Autodesk Inventor part; units mm, degrees
ref_plane "YZ Plane" through (0, 0, 0) normal (1, 0, 0) x (0, 1, 0)
ref_plane "XZ Plane" through (0, 0, 0) normal (0, 1, 0) x (-1, 0, 0)
ref_plane "XY Plane" through (0, 0, 0) normal (0, 0, 1) x (1, 0, 0)
sketch "Sketch1" plane through (0, 0, 0) normal (0, 1, 0) x (-1, 0, 0)
  circle A0 centre (0, 0) radius 12.5
  dimension "d0" = 25
extrude "Extrusion1" add sketch "Sketch1" along normal blind 1
sketch "Sketch2" plane through (0, 1, 0) normal (0, 1, 0) x (1, 0, 0)
  circle A0 centre (0, 0) radius 9.5
  dimension "d3" = 19
extrude "Extrusion2" add sketch "Sketch2" along normal blind 5
sketch "Sketch3" plane through (0, 6, 0) normal (0, 1, 0) x (1, 0, 0)
  circle A0 centre (0, 0) radius 12.5
  dimension "d6" = 25
extrude "Extrusion3" add sketch "Sketch3" along normal blind 1
hole "Hole1" at (-6.2494, 7, 8.9167) direction (0, -1, 0) diameter 1 depth 7
sketch "Sketch4" plane through (0, 7, 0) normal (0, 1, 0) x (1, 0, 0)
  circle A0 centre (0, 0) radius 8.5
  dimension "d18" = 17
extrude "Extrusion4" cut sketch "Sketch4" against normal blind 7
thread "Thread1"
sketch "Sketch5" plane through (0, 0, 0) normal (0, -1, 0) x (1, 0, 0)
  line L0 (11.3779, 4.9373) -> (8.8779, 4.9373)
  line L1 (8.8779, 4.9373) -> (8.8779, -5.0627)
  line L2 (8.8779, -5.0627) -> (11.3779, -5.0627)
  line L3 (11.3779, -5.0627) -> (11.3779, 4.9373)
  point P0 (0, 0)
  dimension "d23" = 10
  dimension "d24" = 2.5
extrude "Extrusion5" add sketch "Sketch5" along normal blind 10
properties part number "Ttube1"
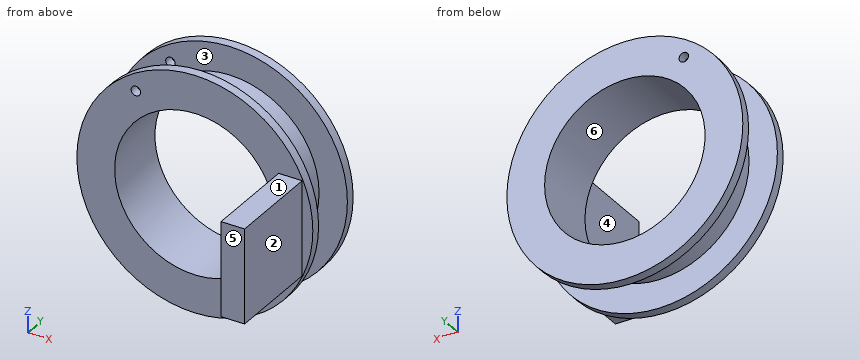
Source: CAD feature listing. Evaluate the final solid. Frame: model axes, mm. Face numbers are marked on the shaded views. A direction names the side the tool comes from. Coordinates: 2 decimals unless noted, no trailing zeros. Order: outer loops, then holes, each group sorted by start corner. A loop starts at its lowest first (then second) coordinate and runs counter-clockwise, first axis right, second up. Notation, with made-up numbers: (16.25, 38) - (63.25, 38) arc R30 ccw to (63.25, 72) - close; hole circle Ø4 at (37.5, -27.75). An arc over 180 degrees is marked (long way). One line per item, written item: value.
1) Cut plane A-A on z = 0. Output: boundary loops of the cut face in (x, y), plus the area to 3 significant figures.
Computed values:
outline: (-12.5, 0) - (-8.5, 0) - (-8.5, 7) - (-12.5, 7) - (-12.5, 6) - (-9.5, 6) - (-9.5, 1) - (-12.5, 1) - close; (8.5, 0) - (8.88, 0) - (8.88, -10) - (11.38, -10) - (11.38, 0) - (12.5, 0) - (12.5, 1) - (9.5, 1) - (9.5, 6) - (12.5, 6) - (12.5, 7) - (8.5, 7) - close
area: 51.0 mm^2
2) Mould query, pull axis X, two halves, no side actions, for the marked faces 4, 5 and 6. Classes: released by +X, released by -X, zero draft, split by the parting line, or undercut.
Computed values:
face 4: released by -X
face 5: zero draft
face 6: undercut
3) Contact query for flat-ended pins moving along their axis: pin 1 (5 mm diameter, centred on x = -6.5, y = -4.5, fed in from -Z); pin 2 (5 mm diameter, centred on x = -6, z = -5.5, fed in from -Y); pin 3 (1.5 mm diameter, centred on x = 6.5, y = 2.5, fed in from +Z); pin 4 (8 mm diameter, centred on y = -7, z = 0.5, fed in from -X). Output: stop coordinate, or through.
Computed values:
pin 1: passes through
pin 2: stops at y = 0
pin 3: stops at z = 7.56
pin 4: stops at x = 8.88
4) Ray query, line 1 (Y direction, x = -10.5, z = 5.5); line 2 (X direction, y = -7.25, z = 1.5); line 3 (Y direction, x = 1.25, z = 8.5). Return the intervals inside material, ascending. Write a range as [from, to].
Computed values:
line 1: y = [0, 1], [6, 7]
line 2: x = [8.88, 11.38]
line 3: y = [0, 7]
5) Cut plane D-D on z = 7. Output: boundary loops of the cut face in (x, y).
Computed values:
outline: (-10.36, 0) - (-4.82, 0) - (-4.82, 7) - (-10.36, 7) - (-10.36, 6) - (-6.42, 6) - (-6.42, 1) - (-10.36, 1) - close; (4.82, 0) - (10.36, 0) - (10.36, 1) - (6.42, 1) - (6.42, 6) - (10.36, 6) - (10.36, 7) - (4.82, 7) - close
6) Reachability of the marked faces 1, 2 and 3 from +Z, -Z, +X, -X, +Y, -Y: full face, straight path, thin tool, end or side. Return the list, or none.
Computed values:
face 1: +Z, +X, -X, -Y
face 2: +Z, -Z, +X, -Y
face 3: none
7) Cut plane C-C on y = 4.5. Output: boundary loops of the cut face in (x, z).
Computed values:
outline: circle Ø19 at (0, 0); hole circle Ø17 at (0, 0)
8) Cut plane B-B on x = 0. Output: boundary loops of the cut face in (y, z).
Computed values:
outline: (0, -12.5) - (1, -12.5) - (1, -9.5) - (6, -9.5) - (6, -12.5) - (7, -12.5) - (7, -8.5) - (0, -8.5) - close; (0, 8.5) - (7, 8.5) - (7, 12.5) - (6, 12.5) - (6, 9.5) - (1, 9.5) - (1, 12.5) - (0, 12.5) - close
